Check sheet for the modelled part. Datum: model origin and axes. Units: mm. A direction names the side the tool comes from. Round coordinates to 2 decimals unless told otherwise and drop trailing zeros. Order: outer loops, then holes, each group sorted by start corner. A loop starts at its lowest first (then second) coordinate and runs counter-clockwise, first axis right, second up.
(1) Tool access check on faces 1 (the flat face through (0, 0, 50)), 2 (the cylindrical face through (-1.894, 14.427, 44.93)). Record the directions out of +Z, -Z, +X, -X, +Y, -Y that give a thin tool (end or side, any length) a straight path to the whole face; none if there is none.
(2) Sectioned sample at B-B, the plane y = -24. Enter the section's corners in (x, z).
(3) Sectioned sample at C-C, the plane z = 26. Enter the section's corners in (x, y).
(4) Thickness scan on probe 1 along Z at (x, y) = (22.5, -13.5); probe 2 along Z at (x, y) = (-38.5, -16); probe 3 along X at (y, z) = (28.5, 14). Record the ranges inside material, lowest first.
(5) Sectioned sample at A-A, the plane x = 0. Enter the section's corners in (y, z).
(6) Depth check by flat-ended pin: pin 1 (8 mm diameter, centred on x = -23.5, y = -46.5, fed in from +Z); pin 2 (2 mm diameter, centred on x = 41, z = 10.5, fed in from +Y); pin 3 (12 mm diameter, centred on y = -29.5, z = 25, fed in from +X). Enter the tip coordinate at first touch or a pass-through.
```python
from build123d import *

# Parameters (mm, degrees)
F0_R     = 60
F1_DEPTH = 30
F2_R     = 30
F3_DEPTH = 10
F4_R     = 14.550501
F5_DEPTH = 10


with BuildPart() as f1:
    # F0 (on Top) → F1 (new body)
    with BuildSketch(Plane.XY):
        Circle(F0_R)
    extrude(amount=F1_DEPTH)

    # F2 (on face) → F3 (join)
    with BuildSketch(Plane.XY.offset(30)):
        Circle(F2_R)
    extrude(amount=F3_DEPTH)

    # F4 (on face) → F5 (join)
    with BuildSketch(Plane.XY.offset(40)):
        Circle(F4_R)
    extrude(amount=F5_DEPTH)


solid = f1.part
```
Derived:
1. face 1: +Z, +X, -X, +Y, -Y
1. face 2: +Z
2. outline: (-54.99, 0) - (54.99, 0) - (54.99, 30) - (18, 30) - (18, 40) - (-18, 40) - (-18, 30) - (-54.99, 30) - close
3. outline: circle Ø120 at (0, 0)
4. probe 1: z = 0 to 40
4. probe 2: z = 0 to 30
4. probe 3: x = -52.8 to 52.8
5. outline: (-60, 0) - (60, 0) - (60, 30) - (30, 30) - (30, 40) - (14.55, 40) - (14.55, 50) - (-14.55, 50) - (-14.55, 40) - (-30, 40) - (-30, 30) - (-60, 30) - close
6. pin 1: stops at z = 30
6. pin 2: stops at y = 44.72
6. pin 3: stops at x = 55.21
